Can you work these out from the model? Positions are in its coordinate system, mm. Face numbers are marked on the shaded views. A direction names the side the tool comes from. Coordinates: 2 decimals unless noted, no trailing zeros. Loops run counter-clockwise (first coordinate to the right, second up) from the corner with the lowest first, then second, coordinate; pieces in that order, holes last. Notation, with made-up numbers: (48, -38.75) -> (89, -38.75) arc R18 ccw to (89, -7.75) -> close; hole circle Ø9 at (66.25, -2). An arc over 180 degrees is marked (long way). Put each result on its own line as item: value. Start each with the question number.
Item 1: If we section it at B-B on x = 19.7: Please give me the cut outline in (y, z).
Item 2: We'd pull the mould along X, two halves only. Please class the marked faces 3, 4 and 5: pulls with the +X half, pulls with the -X half, needs draft (parallel to the pull), parting line crosses it, or undercut.
Item 3: If we section it at A-A on x = 3.3: Please give me the cut outline in (y, z), plus the area to 3 significant figures.
Item 4: If we section it at C-C on z = 11.5: Please give me the cut outline in (x, y).
Item 5: For the marked faces 1 and 2, which set-ups out of +Z, -Z, +X, -X, +Y, -Y let a thin tool reach every point of the face, with its end or its side?
Item 6: If we section it at D-D on y = 2.8: Please give me the cut outline in (x, z).
Item 7: Will these pins go through, and if not, where does the flat tip stop? P1, Ø0.9, axis at x = 20.5, y = 3, coming from the +Z side; P2, Ø0.9, axis at x = -6, y = 0.5, coming from the +Z side; P3, Ø2, axis at x = 2, z = 15.5, coming from the +Y side; P4, Ø1, axis at x = 11.5, y = 1, coming from the -Z side.
Item 8: Please list where these lines run through material, in increasing order: L1, parallel to Z at x = 3.3, y = 0.35; L2, parallel to Z at x = 19.7, y = 0.2; L3, parallel to Y at x = 4.5, z = 1.5. Write a range as from..to.
```python
from build123d import *

# Parameters (mm, degrees)
SKETCH1_R           = 0.5
BOSS_EXTRUDE1_DEPTH = 0.83
SKETCH2_W           = 4.5
SKETCH2_H           = 6
BOSS_EXTRUDE2_DEPTH = 3


with BuildPart() as part:
    # Sketch1 → Boss-Extrude1 (new body)
    with BuildSketch(Plane(origin=(0, 0, 0), x_dir=(1, 0, 0), z_dir=(0, 1, 0))):
        Polygon((0, 0), (-2.83, -3.2), (-7, -3.2), (-7, -16.8), (-3, -16.8), (0, -20), (23, -20), (23, 0), align=None)
        with Locations((3.3, -18.217292277)):
            Circle(SKETCH1_R, mode=Mode.SUBTRACT)
        with Locations((3.3, -1.817292277)):
            Circle(SKETCH1_R, mode=Mode.SUBTRACT)
        with Locations((19.7, -18.217292277)):
            Circle(SKETCH1_R, mode=Mode.SUBTRACT)
    extrude(amount=BOSS_EXTRUDE1_DEPTH)

    # Sketch2 → Boss-Extrude2 (add)
    with BuildSketch(Plane(origin=(0, 0.83, 0), x_dir=(1, 0, 0), z_dir=(0, 1, 0))):
        with Locations((20.75, -10)):
            Rectangle(SKETCH2_W, SKETCH2_H)
    extrude(amount=BOSS_EXTRUDE2_DEPTH)


solid = part.part
```
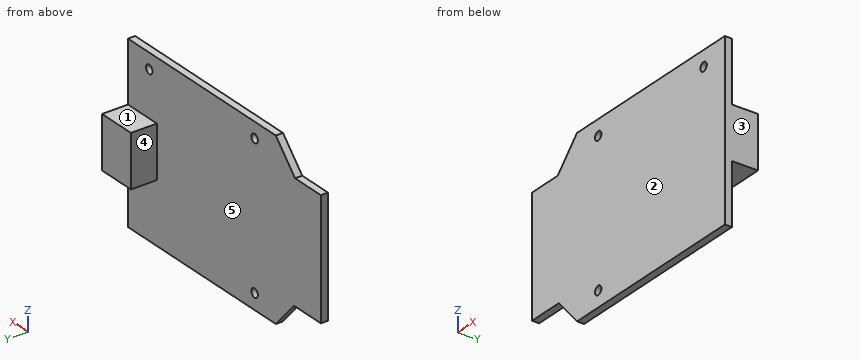
Solutions:
1. outline: (0, 0) -> (0.83, 0) -> (0.83, 7) -> (3.83, 7) -> (3.83, 13) -> (0.83, 13) -> (0.83, 17.72) -> (0, 17.72) -> close; (0, 18.72) -> (0.83, 18.72) -> (0.83, 20) -> (0, 20) -> close
2. face 3: pulls with the +X half
2. face 4: pulls with the -X half
2. face 5: needs draft
3. outline: (0, 0) -> (0.83, 0) -> (0.83, 1.32) -> (0, 1.32) -> close; (0, 2.32) -> (0.83, 2.32) -> (0.83, 17.72) -> (0, 17.72) -> close; (0, 18.72) -> (0.83, 18.72) -> (0.83, 20) -> (0, 20) -> close
3. area: 14.9 mm^2
4. outline: (-7, 0) -> (23, 0) -> (23, 3.83) -> (18.5, 3.83) -> (18.5, 0.83) -> (-7, 0.83) -> close
5. face 1: +Z, +X, -X, +Y
5. face 2: +Z, -Z, +X, -X, -Y
6. outline: (18.5, 7) -> (23, 7) -> (23, 13) -> (18.5, 13) -> close
7. P1: z = 13
7. P2: z = 16.8
7. P3: y = 0.83
7. P4: z = 0
8. L1: 0..1.32, 2.32..17.72, 18.72..20
8. L2: 0..17.72, 18.72..20
8. L3: 0..0.83
